from build123d import *

# Parameters (mm, degrees)
SKETCH1_W                 = 75
SKETCH1_H                 = 40
SKETCH1_R                 = 5
SKETCH1_R_2               = 1.7
SKETCH1_R_3               = 1.197563381
SKETCH1_W_2               = 5
SKETCH1_H_2               = 20
BOSS_EXTRUDE1_DEPTH       = 3
CUT_EXTRUDE1_DEPTH        = 43.605750786
CUT_EXTRUDE1_DEPTH_BACK   = 43.605750786
SKETCH2_W                 = 67
SKETCH2_H                 = 28
BOSS_EXTRUDE3_DEPTH       = 90
BOSS_EXTRUDE3_DEPTH_BACK  = 3
SKETCH6_W                 = 67
SKETCH6_H                 = 11
CUT_EXTRUDE4_DEPTH        = 104.591746776
SKETCH7_W                 = 70
SKETCH7_H                 = 37
BOSS_EXTRUDE4_DEPTH       = 45
SKETCH8_W                 = 45
SKETCH8_H                 = 62
CUT_EXTRUDE6_DEPTH        = 29
SKETCH11_W                = 45
SKETCH11_H                = 4
CUT_EXTRUDE9_DEPTH        = 143.671826231
SKETCH9_W                 = 38
SKETCH9_H                 = 28.5
CUT_EXTRUDE10_DEPTH       = 193.611006954
SKETCH13_W                = 5
SKETCH13_H                = 38
BOSS_EXTRUDE5_DEPTH       = 32
SKETCH14_R                = 5
SKETCH14_R_2              = 1.7
CUT_EXTRUDE11_DEPTH       = 32
SKETCH15_W                = 165
SKETCH15_H                = 70
SKETCH15_W_2              = 157
SKETCH15_H_2              = 62
BOSS_EXTRUDE6_DEPTH       = 3
SKETCH16_W                = 20
SKETCH16_H                = 4.820648258
CUT_EXTRUDE12_DEPTH       = 145.645255712
SKETCH18_R                = 5
CUT_EXTRUDE14_DEPTH       = 145.645255712
MIRROR6_COPY_1_SKETCH_W   = 5
MIRROR6_COPY_1_SKETCH_H   = 38
MIRROR6_COPY_1_DEPTH      = 32
MIRROR6_COPY_2_SKETCH_R   = 5
MIRROR6_COPY_2_SKETCH_R_2 = 1.7
MIRROR6_COPY_2_DEPTH      = 32
SKETCH19_W                = 38
SKETCH19_H                = 3.5
CUT_EXTRUDE15_DEPTH       = 10


with BuildPart() as part:
    # Sketch1 → Boss-Extrude1 (new body)
    with BuildSketch(Plane(origin=(0, 0, 0), x_dir=(1, 0, 0), z_dir=(0, 1, 0))):
        Rectangle(SKETCH1_W, SKETCH1_H)
        with Locations(Location((-21, 0, 0), (0, 0, 270))):
            Circle(SKETCH1_R, mode=Mode.SUBTRACT)
        with Locations(Location((-30, 8.25, 0), (0, 0, 270))):
            Circle(SKETCH1_R_2, mode=Mode.SUBTRACT)
        with Locations(Location((-12, 8.25, 0), (0, 0, 270))):
            Circle(SKETCH1_R_2, mode=Mode.SUBTRACT)
        with Locations(Location((-12, -8.25, 0), (0, 0, 270))):
            Circle(SKETCH1_R_2, mode=Mode.SUBTRACT)
        with Locations(Location((-30, -8.25, 0), (0, 0, 270))):
            Circle(SKETCH1_R_2, mode=Mode.SUBTRACT)
        with Locations(Location((12, 8.25, 0), (0, 0, 90))):
            Circle(SKETCH1_R_2, mode=Mode.SUBTRACT)
        with Locations(Location((12, -8.25, 0), (0, 0, 90))):
            Circle(SKETCH1_R_2, mode=Mode.SUBTRACT)
        with Locations(Location((21, 0, 0), (0, 0, 90))):
            Circle(SKETCH1_R, mode=Mode.SUBTRACT)
        with Locations(Location((30, -8.25, 0), (0, 0, 90))):
            Circle(SKETCH1_R_2, mode=Mode.SUBTRACT)
        with Locations(Location((30, 8.25, 0), (0, 0, 90))):
            Circle(SKETCH1_R_2, mode=Mode.SUBTRACT)
        with Locations(Location((-30, -17.5, 0), (0, 0, 270))):
            Circle(SKETCH1_R_3, mode=Mode.SUBTRACT)
        with Locations(Location((-12, -17.5, 0), (0, 0, 270))):
            Circle(SKETCH1_R_3, mode=Mode.SUBTRACT)
        with Locations(Location((12, -17.5, 0), (0, 0, 90))):
            Circle(SKETCH1_R_3, mode=Mode.SUBTRACT)
        with Locations(Location((30, -17.5, 0), (0, 0, 90))):
            Circle(SKETCH1_R_3, mode=Mode.SUBTRACT)
        with Locations(Location((30, 17.5, 0), (0, 0, 270))):
            Circle(SKETCH1_R_3, mode=Mode.SUBTRACT)
        with Locations(Location((12, 17.5, 0), (0, 0, 270))):
            Circle(SKETCH1_R_3, mode=Mode.SUBTRACT)
        with Locations(Location((-12, 17.5, 0), (0, 0, 90))):
            Circle(SKETCH1_R_3, mode=Mode.SUBTRACT)
        with Locations(Location((-30, 17.5, 0), (0, 0, 90))):
            Circle(SKETCH1_R_3, mode=Mode.SUBTRACT)
        Rectangle(SKETCH1_W_2, SKETCH1_H_2, mode=Mode.SUBTRACT)
    extrude(amount=BOSS_EXTRUDE1_DEPTH)

    # Sketch2 → Cut-Extrude1 (cut, two sides: drawn at the far end of the back side and taken through both)
    with BuildSketch(Plane(origin=(0, 3, 0), x_dir=(1, 0, 0), z_dir=(0, 1, 0)).offset(-CUT_EXTRUDE1_DEPTH_BACK)):
        Rectangle(SKETCH2_W, SKETCH2_H)
    extrude(amount=CUT_EXTRUDE1_DEPTH + CUT_EXTRUDE1_DEPTH_BACK, mode=Mode.SUBTRACT)

    # Sketch3 → Boss-Extrude3 (add, two sides: drawn at the far end of the back side and taken through both)
    with BuildSketch(Plane(origin=(0, 3, 0), x_dir=(1, 0, 0), z_dir=(0, 1, 0)).offset(-BOSS_EXTRUDE3_DEPTH_BACK)):
        Polygon((37.5, -35), (37.5, -20), (33.5, -20), (-33.5, -20), (-37.5, -20), (-37.5, -35), align=None)
        Polygon((33.5, 20), (37.5, 20), (37.5, 35), (-37.5, 35), (-37.5, 20), (-33.5, 20), align=None)
        Polygon((37.5, -20), (37.5, 20), (33.5, 20), (33.5, 14), (33.5, -14), (33.5, -20), align=None)
        Polygon((-33.5, 14), (-33.5, 20), (-37.5, 20), (-37.5, -20), (-33.5, -20), (-33.5, -14), align=None)
    extrude(amount=BOSS_EXTRUDE3_DEPTH + BOSS_EXTRUDE3_DEPTH_BACK)

    # Sketch6 → Cut-Extrude4 (cut, through all)
    with BuildSketch(Plane(origin=(0, 3, 0), x_dir=(1, 0, 0), z_dir=(0, 1, 0))):
        with Locations((0, -25.5)):
            Rectangle(SKETCH6_W, SKETCH6_H)
        with Locations((0, 25.5)):
            Rectangle(SKETCH6_W, SKETCH6_H)
    extrude(amount=CUT_EXTRUDE4_DEPTH, mode=Mode.SUBTRACT)

    # Sketch7 → Boss-Extrude4 (add)
    with BuildSketch(Plane.ZY.offset(37.5)):
        with Locations((0, 74.5)):
            Rectangle(SKETCH7_W, SKETCH7_H)
    boss_extrude4 = extrude(amount=BOSS_EXTRUDE4_DEPTH)

    # Mirror2: Boss-Extrude4 across plane
    add(boss_extrude4.mirror(Plane(origin=(0, 0, 0), x_dir=(0, 0, 1), z_dir=(1, 0, 0))))

    # Sketch8 → Cut-Extrude6 (cut)
    with BuildSketch(Plane(origin=(0, 93, 0), x_dir=(1, 0, 0), z_dir=(0, 1, 0))):
        with Locations((-56, 0)):
            Rectangle(SKETCH8_W, SKETCH8_H)
        with Locations((56, 0)):
            Rectangle(SKETCH8_W, SKETCH8_H)
    extrude(amount=-CUT_EXTRUDE6_DEPTH, mode=Mode.SUBTRACT)

    # Sketch11 → Cut-Extrude9 (cut, through all)
    with BuildSketch(Plane.XY.offset(35)):
        with Locations((-60, 58)):
            Rectangle(SKETCH11_W, SKETCH11_H)
        with Locations((60, 58)):
            Rectangle(SKETCH11_W, SKETCH11_H)
    extrude(amount=-CUT_EXTRUDE9_DEPTH, mode=Mode.SUBTRACT)

    # Sketch9 → Cut-Extrude10 (cut, through all)
    with BuildSketch(Plane.ZY.offset(82.5)):
        with Locations((0, 78.25)):
            Rectangle(SKETCH9_W, SKETCH9_H)
    extrude(amount=-CUT_EXTRUDE10_DEPTH, mode=Mode.SUBTRACT)

    # Sketch13 → Boss-Extrude5 (add)
    with BuildSketch(Plane(origin=(0, 64, 0), x_dir=(1, 0, 0), z_dir=(0, 1, 0))):
        with Locations((-54.5, 0)):
            Rectangle(SKETCH13_W, SKETCH13_H)
    boss_extrude5 = extrude(amount=BOSS_EXTRUDE5_DEPTH)

    # Sketch14 → Cut-Extrude11 (cut)
    with BuildSketch(Plane.ZY.offset(57)):
        with Locations((0, 78.25)):
            Circle(SKETCH14_R)
        with Locations((-9, 86.202083543)):
            Circle(SKETCH14_R_2)
        with Locations((9, 86.202083543)):
            Circle(SKETCH14_R_2)
        with Locations((9, 69.702083543)):
            Circle(SKETCH14_R_2)
        with Locations((-9, 69.702083543)):
            Circle(SKETCH14_R_2)
    cut_extrude11 = extrude(amount=-CUT_EXTRUDE11_DEPTH, mode=Mode.SUBTRACT)

    # Mirror4: Boss-Extrude5, Cut-Extrude11 across plane
    add(boss_extrude5.mirror(Plane(origin=(0, 0, 0), x_dir=(0, 0, 1), z_dir=(1, 0, 0))))
    add(cut_extrude11.mirror(Plane(origin=(0, 0, 0), x_dir=(0, 0, 1), z_dir=(1, 0, 0))), mode=Mode.SUBTRACT)

    # Sketch15 → Boss-Extrude6 (add)
    with BuildSketch(Plane(origin=(0, 93, 0), x_dir=(1, 0, 0), z_dir=(0, 1, 0))):
        Rectangle(SKETCH15_W, SKETCH15_H)
        Rectangle(SKETCH15_W_2, SKETCH15_H_2, mode=Mode.SUBTRACT)
    extrude(amount=BOSS_EXTRUDE6_DEPTH)

    # Sketch16 → Cut-Extrude12 (cut, through all)
    with BuildSketch(Plane.XY.offset(35)):
        with Locations((0, 11.636111214)):
            Rectangle(SKETCH16_W, SKETCH16_H)
    extrude(amount=-CUT_EXTRUDE12_DEPTH, mode=Mode.SUBTRACT)

    # Sketch18 → Cut-Extrude14 (cut, through all)
    with BuildSketch(Plane.XY.offset(35)):
        with Locations((67.75, 80)):
            Circle(SKETCH18_R)
    cut_extrude14 = extrude(amount=-CUT_EXTRUDE14_DEPTH, mode=Mode.SUBTRACT)

    # Mirror5: Cut-Extrude14 across plane
    add(cut_extrude14.mirror(Plane(origin=(0, 0, 0), x_dir=(0, 0, 1), z_dir=(1, 0, 0))), mode=Mode.SUBTRACT)

    # Mirror6: Boss-Extrude5, Cut-Extrude11 across plane
    add(boss_extrude5.mirror(Plane.ZX.offset(96)))
    add(cut_extrude11.mirror(Plane.ZX.offset(96)), mode=Mode.SUBTRACT)

    # Mirror6 copy 1 sketch → Mirror6 copy 1 (add)
    with BuildSketch(Plane(origin=(0, 128, 0), x_dir=(-1, 0, 0), z_dir=(0, -1, 0))):
        with Locations((-54.5, 0)):
            Rectangle(MIRROR6_COPY_1_SKETCH_W, MIRROR6_COPY_1_SKETCH_H)
    extrude(amount=MIRROR6_COPY_1_DEPTH)

    # Mirror6 copy 2 sketch → Mirror6 copy 2 (cut)
    with BuildSketch(Plane(origin=(57, 192, 0), x_dir=(0, 0, 1), z_dir=(1, 0, 0))):
        with Locations((0, 78.25)):
            Circle(MIRROR6_COPY_2_SKETCH_R)
        with Locations((-9, 86.202083543)):
            Circle(MIRROR6_COPY_2_SKETCH_R_2)
        with Locations((9, 86.202083543)):
            Circle(MIRROR6_COPY_2_SKETCH_R_2)
        with Locations((9, 69.702083543)):
            Circle(MIRROR6_COPY_2_SKETCH_R_2)
        with Locations((-9, 69.702083543)):
            Circle(MIRROR6_COPY_2_SKETCH_R_2)
    extrude(amount=-MIRROR6_COPY_2_DEPTH, mode=Mode.SUBTRACT)

    # Sketch19 → Cut-Extrude15 (cut)
    with BuildSketch(Plane(origin=(82.5, 0, 0), x_dir=(0, 0, -1), z_dir=(1, 0, 0))):
        with Locations((0, 94.25)):
            Rectangle(SKETCH19_W, SKETCH19_H)
    cut_extrude15 = extrude(amount=-CUT_EXTRUDE15_DEPTH, mode=Mode.SUBTRACT)

    # Mirror7: Cut-Extrude15 across plane
    add(cut_extrude15.mirror(Plane(origin=(0, 0, 0), x_dir=(0, 0, 1), z_dir=(1, 0, 0))), mode=Mode.SUBTRACT)


solid = part.part
Work out the finished part from the listing and answer in its coordinate system (mm). A direction names the side the tool comes from. Round coordinates to 2 decimals unless told otherwise and drop trailing zeros. Order: outer loops, then holes, each group sorted by start corner. A loop starts at its lowest first (then second) coordinate and runs counter-clockwise, first axis right, second up. Notation, with made-up numbers: M 60.25,62 L 94.25,62 A19 cw 94.25,88 Z; hole C 20,16 d9. An arc over 180 degrees is marked long. Put each result on its own line as item: value. Start each with the question number.
Q1. Straight lines are drawn through the part: L1, parallel to Y at x = 54.95, z = 0; L2, parallel to X at y = 30, z = 17; L3, parallel to X at y = 93, z = -29.5. For each, find the intervals that lie inside material, in ascending order. Write a range as [from, to].
Q2. Section A-A, the plane x = 67.75 is taken. Write down the section's boundary in (y, z).
Q3. Section C-C, the plane x = 15.5 is taken. Write down the section's boundary in (y, z).
Q4. For a pull along Y with two mould halves and no side action, classify faces 5 (the flat face through (-78.5, 80, -25)), 6 (the flat face through (0, 14.046, 33)), 7 (the flat face through (0, 3, -23)) as pulls with the +Y half, pulls with the -Y half, needs draft (parallel to the pull), parting line crosses it, or undercut.
Q5. Section D-D, the plane y = 40.5 is taken. Write down the section's boundary in (x, z), and give its area (3 significant figures).
Q6. Flat-ended cylindrical pins translate along their axes: pin 1 (5.5 mm diameter, centred on y = 86.2, z = 9, fed in from +X); pin 2 (5 mm diameter, centred on x = -29.5, z = 23.5, fed in from +Y); pin 3 (1 mm diameter, centred on x = -35.5, z = -26, fed in from -Y); pin 4 (11.5 mm diameter, centred on y = 78.25, z = 0, fed in from -X). Find the tip coordinate at first contact, or state that the pin passes through.
Q7. Section B-B, the plane y = 113.75 is taken. Write down the section's boundary in (x, z), and give its area (3 significant figures).
Q8. A tool of negligible diameter and unlimited length cuts with its end or side. For faces 1 (the flat face through (-81, 80, 19)), 2 (the flat face through (-33.5, 32, 0)), 3 (the flat face through (80, 80, 19)), 4 (the flat face through (10, 12, -33)), from which of +Z, -Z, +X, -X, +Y, -Y can it reach the whole face along a straight path? Write none if from no direction.
Findings below:
1. L1: y = [60, 73.25], [83.25, 108.75], [118.75, 128]
1. L2: x = [-37.5, -33.5], [33.5, 37.5]
1. L3: x = [-82.5, -78.5], [78.5, 82.5]
2. outline: M 60,-35 L 75,-35 L 75,-31 L 64,-31 L 64,31 L 75,31 L 75,35 L 60,35 Z; M 85,-35 L 96,-35 L 96,-31 L 85,-31 Z; M 85,31 L 96,31 L 96,35 L 85,35 Z
3. outline: M 0,-35 L 96,-35 L 96,-31 L 3,-31 L 3,-14 L 0,-14 Z; M 0,14 L 3,14 L 3,31 L 96,31 L 96,35 L 0,35 Z
4. face 5: needs draft
4. face 6: undercut
4. face 7: pulls with the +Y half
5. outline: M -37.5,-35 L 37.5,-35 L 37.5,35 L -37.5,35 Z; hole M -33.5,-31 L 33.5,-31 L 33.5,31 L -33.5,31 Z
5. area: 1,100 mm^2
6. pin 1: stops at x = 57
6. pin 2: stops at y = 3
6. pin 3: stops at y = 0
6. pin 4: stops at x = -57
7. outline: M -57,-19 L -52,-19 L -52,-5 L -57,-5 Z; M -57,5 L -52,5 L -52,19 L -57,19 Z; M 52,-19 L 57,-19 L 57,-5 L 52,-5 Z; M 52,5 L 57,5 L 57,19 L 52,19 Z
7. area: 280 mm^2
8. face 1: -X, +Y
8. face 2: +Y
8. face 3: +X, +Y
8. face 4: +Z, -Z
